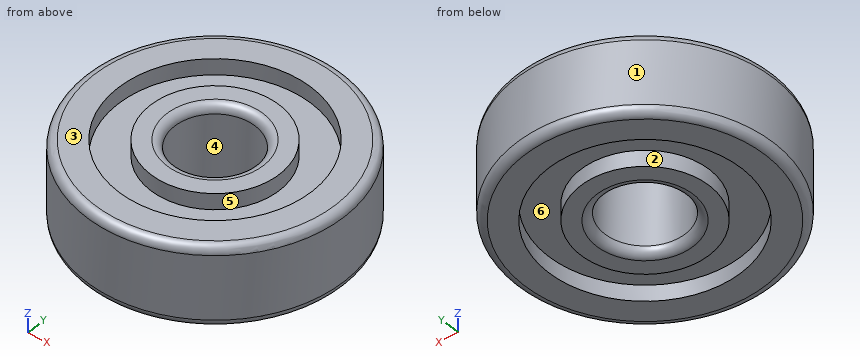
from build123d import *

# Parameters (mm, degrees)
SKETCH_3_R          = 8
SKETCH_3_R_2        = 2.5
EXTRUDE_1_DEPTH     = 2.5
FILLET_1_R          = 0.5
SKETCH_4_R          = 6
SKETCH_4_R_2        = 4
CUT_EXTRUDE_1_DEPTH = 1


with BuildPart() as part:
    # 草圖3 → 填料-伸長1 (new, symmetric)
    with BuildSketch(Plane.XY):
        Circle(SKETCH_3_R)
        Circle(SKETCH_3_R_2, mode=Mode.SUBTRACT)
    extrude(amount=EXTRUDE_1_DEPTH, both=True)

    # 圓角1
    fillet_1_edges = [part.edges().sort_by_distance(p)[0] for p in [
        (-8, 0, -2.5),
        (-8, 0, 2.5),
        (-2.5, 0, -2.5),
        (-2.5, 0, 2.5),
    ]]
    fillet(fillet_1_edges, radius=FILLET_1_R)

    # 草圖4 → 除料-伸長1 (cut)
    with BuildSketch(Plane(origin=(0, 0, -2.5), x_dir=(-1, 0, 0), z_dir=(0, 0, -1))):
        Circle(SKETCH_4_R)
        Circle(SKETCH_4_R_2, mode=Mode.SUBTRACT)
    cut_extrude_1 = extrude(amount=-CUT_EXTRUDE_1_DEPTH, mode=Mode.SUBTRACT)

    # 鏡射1: 除料-伸長1 across plane
    add(cut_extrude_1.mirror(Plane.XY), mode=Mode.SUBTRACT)


solid = part.part
CAD build for the part. Positions are in the model's coordinates, mm. Face numbers are marked on the shaded views. A direction names the side the tool comes from. Coordinates: 2 decimals unless noted, no trailing zeros. Write each loop counter-clockwise with the first axis right and the second up, starting at its lowest first coordinate (ties: lowest second). Pieces come first, ordered by that corner, then holes. Notation, with made-up numbers: M 31.5,65 L 46.5,65 A27 cw 46.5,95 Z; hole C -23.5,-14 d5. An arc over 180 degrees is marked long. Answer as a JSON object with one key per item and string values. Group by question number.
1) Mould opens along Y. For the marked faces 1, 2 and 3 say: +Y half, -Y half, draft (parallel to the pull), parting line (faces both ways), or undercut.
2) Saw through at C-C (z = -0.5). Write the cut outline in (x, y).
3) Tool access for the marked faces 4, 5 and 6: list every direction of +Z, -Z, +X, -X, +Y, -Y with a clear straight run to the whole face (end or side of a thin tool).
4) Wall check: line 1 (Y direction, x = 0, z = 1.8); line 2 (Y direction, x = 0, z = -0.45); line 3 (Z direction, x = -4.5, y = -0.25). Give the ranges that are in metal, low to high. Write a range as from..to.
5) Pin check, flat tip, straight feed: pin 1 Ø1.5 at (y, z) = (-1.5, -1) entering from -X. Stop position of the tip, or through.
Values follow:
{
 "1": {"face 1": "parting line", "face 2": "undercut", "face 3": "draft"},
 "2": {"outline": "C 0,0 d16; hole C 0,0 d5"},
 "3": {"face 4": "+Z, -Z", "face 5": "+Z", "face 6": "-Z"},
 "4": {"line 1": "y = -8..-6, -4..-2.5, 2.5..4, 6..8", "line 2": "y = -8..-2.5, 2.5..8", "line 3": "z = -1.5..1.5"},
 "5": {"pin 1": "stops at x = -7.96"}
}
